Input: dimensioned drawing with shaded views. Units: mm. Origin: part minimum x, y, z. Give positions to 0.01 mm unless a question says otherwise; leave off trailing zeros. Loops run counter-clockwise (first coordinate to the right, second up) from the corner with the lowest first, then second, coordinate; pieces in that order, holes last.
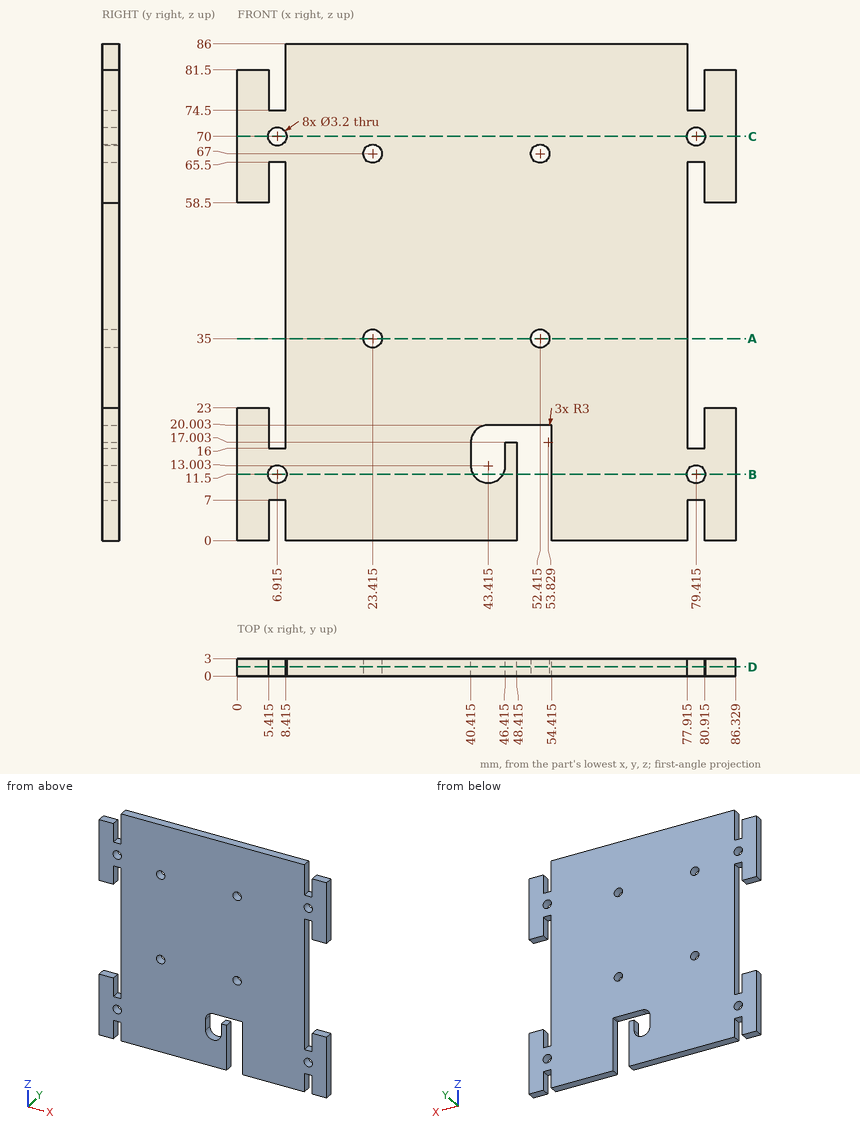
Item 1: Section query A-A on z = 35. Return loops of the section in (x, y) (1 decimal), plus the area to 3 significant figures.
Values follow:
outline: (8.4, 0) - (21.8, 0) - (21.8, 3) - (8.4, 3) - close; (25, 0) - (50.8, 0) - (50.8, 3) - (25, 3) - close; (54, 0) - (77.9, 0) - (77.9, 3) - (54, 3) - close
area: 189 mm2
Item 2: Pin query (flat end, axial travel): pin 1 (1.5 mm diameter, centred on x = 2, y = 1, fed in from +Z); pin 2 (5 mm diameter, centred on x = 52.41, z = 35, fed in from +Y); pin 3 (1 mm diameter, centred on y = 1, z = 39.5, fed in from -X) (1 decimal); pin 4 (1.5 mm diameter, centred on x = 79, y = 1, fed in from +Z). Return the tip coordinate at first contact, or that it passes through.
Values follow:
pin 1: stops at z = 81.5
pin 2: stops at y = 3
pin 3: stops at x = 8.4
pin 4: stops at z = 74.5
Item 3: Ray query, probe 1 along X at (y, z) = (0.6, 22.5) (1 decimal); probe 2 along X at (y, z) = (0.6, 35) (1 decimal); probe 3 along Z at (x, y) = (7, 1.1). Return the intervals inside material, ascending.
Values follow:
probe 1: x = 0 to 5.4, 8.4 to 77.9, 80.9 to 86.3
probe 2: x = 8.4 to 21.8, 25 to 50.8, 54 to 77.9
probe 3: z = 7 to 9.9, 13.1 to 16, 65.5 to 68.4, 71.6 to 74.5
Item 4: Section query D-D on y = 1.6. Give the number of separate pieces and of enclosed holes in the cut face, plus the area to 3 significant figures.
Values follow:
separate pieces: 1
enclosed holes: 8
area: 6,340 mm2
Item 5: Section query C-C on z = 70. Return loops of the section in (x, y) (1 decimal), plus the area to 3 significant figures.
Values follow:
outline: (0, 0) - (5.3, 0) - (5.3, 3) - (0, 3) - close; (8.5, 0) - (77.8, 0) - (77.8, 3) - (8.5, 3) - close; (81, 0) - (86.3, 0) - (86.3, 3) - (81, 3) - close
area: 240 mm2
Item 6: Section query B-B on z = 11.5. Return loops of the section in (x, y) (1 decimal).
Values follow:
outline: (0, 0) - (5.3, 0) - (5.3, 3) - (0, 3) - close; (8.5, 0) - (40.8, 0) - (40.8, 3) - (8.5, 3) - close; (46, 0) - (48.4, 0) - (48.4, 3) - (46, 3) - close; (54.4, 0) - (77.8, 0) - (77.8, 3) - (54.4, 3) - close; (81, 0) - (86.3, 0) - (86.3, 3) - (81, 3) - close
